from build123d import *

# Parameters (mm, degrees)
SKETCH1_R           = 1.5875
SKETCH1_R_2         = 1.905
SKETCH1_R_3         = 13.5001
BOSS_EXTRUDE1_DEPTH = 6.35


with BuildPart() as part:
    # Sketch1 → Boss-Extrude1 (new body)
    with BuildSketch(Plane.XY):
        with BuildLine():
            ThreePointArc((17.78, 25.4), (18.678025612, 25.028025612), (19.05, 24.13))
            Line((19.05, 24.13), (19.05, 0))
            ThreePointArc((19.05, 0), (13.470384182, -13.470384182), (0, -19.05))
            Line((0, -19.05), (-26.67, -19.05))
            ThreePointArc((-26.67, -19.05), (-67.081152545, -2.311152545), (-83.82, 38.1))
            ThreePointArc((-83.82, 38.1), (-81.588153673, 43.488153673), (-76.2, 45.72))
            Line((-76.2, 45.72), (-50.8, 45.72))
            ThreePointArc((-50.8, 45.72), (-47.214117647, 44.823529412), (-44.471972318, 42.345051903))
            ThreePointArc((-44.471972318, 42.345051903), (-30.704117647, 29.901029412), (-12.7, 25.4))
            Line((-12.7, 25.4), (17.78, 25.4))
        make_face()
        with Locations((-7.750175, 13.423696868)):
            Circle(SKETCH1_R, mode=Mode.SUBTRACT)
        with Locations((-13.423696868, 7.750175)):
            Circle(SKETCH1_R, mode=Mode.SUBTRACT)
        with Locations((-15.50035, 0)):
            Circle(SKETCH1_R, mode=Mode.SUBTRACT)
        with Locations((-13.423696868, -7.750175)):
            Circle(SKETCH1_R, mode=Mode.SUBTRACT)
        with Locations((-7.750175, -13.423696868)):
            Circle(SKETCH1_R, mode=Mode.SUBTRACT)
        with Locations((0, -15.50035)):
            Circle(SKETCH1_R, mode=Mode.SUBTRACT)
        with Locations((7.750175, -13.423696868)):
            Circle(SKETCH1_R, mode=Mode.SUBTRACT)
        with Locations((13.423696868, -7.750175)):
            Circle(SKETCH1_R, mode=Mode.SUBTRACT)
        with Locations((15.50035, 0)):
            Circle(SKETCH1_R, mode=Mode.SUBTRACT)
        with Locations((13.423696868, 7.750175)):
            Circle(SKETCH1_R, mode=Mode.SUBTRACT)
        with Locations((7.750175, 13.423696868)):
            Circle(SKETCH1_R, mode=Mode.SUBTRACT)
        with Locations((0, 15.50035)):
            Circle(SKETCH1_R, mode=Mode.SUBTRACT)
        with Locations((-50.8, 38.1)):
            Circle(SKETCH1_R_2, mode=Mode.SUBTRACT)
        with Locations((-76.2, 38.1)):
            Circle(SKETCH1_R_2, mode=Mode.SUBTRACT)
        Circle(SKETCH1_R_3, mode=Mode.SUBTRACT)
    extrude(amount=BOSS_EXTRUDE1_DEPTH)


solid = part.part
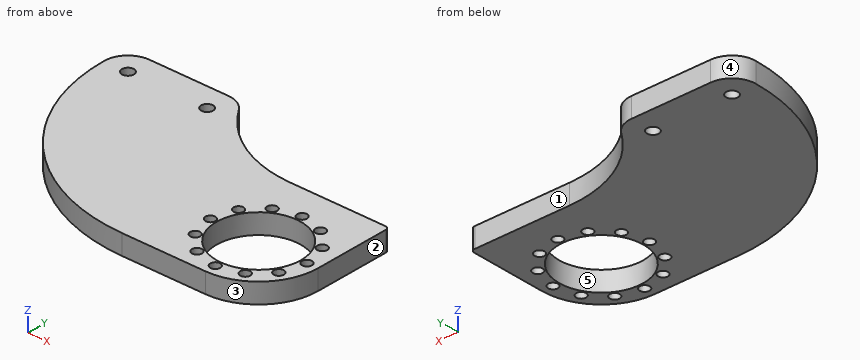
Model file for the job. Use its own axes, mm. Face numbers are marked on the shaded views. A direction names the side the tool comes from. Coordinates: 2 decimals unless noted, no trailing zeros. Write each loop counter-clockwise with the first axis right and the second up, starting at its lowest first coordinate (ties: lowest second). Pieces come first, ordered by that corner, then holes. Notation, with made-up numbers: (48.25, -33.5) -> (83.25, -33.5) arc R19 ccw to (83.25, -28.5) -> close; hole circle Ø5 at (-2, 2.25). An arc over 180 degrees is marked (long way). One line per item, written item: value. Start each with the question number.
1) Pull direction X, two halves, no side cores. Call the marked faces 3, 4 and 5: +X half, -X half, draft (parallel to the pull), parting line (faces both ways), or undercut.
2) Probe probe 1 along Y at (x, z) = (-7, 5.5); probe 2 along Y at (x, z) = (-1, 3.75); probe 3 along X at (y, z) = (38, 5). List the from-to ranges inside material, lowest first.
3) Slice it at C-C on y = 19.5. Write the cut outline in (x, z).
4) Slice it at B-B on z = 2.5. Count the separate pieces of the cut face and the enclosed holes in it, then the cut area to 3 significant figures.
5) Which spindle directions (+Z, -Z, +X, -X, +Y, -Y) get a long thin tool onto all of the face, cutting with end or side? Do the marked faces 1 and 2. Say none if no direction does.
6) Flat gauge pins, fed straight in: pin 1 Ø2 at (y, z) = (-7, 3.5) entering from -X; pin 2 Ø24.5 at (x, y) = (0, 0) entering from -Z; pin 3 Ø3 at (x, z) = (5, 3) entering from +Y. Where does each tip first touch, or does it go through?
7) Slice it at A-A on x = 5. Write the cut outline in (y, z).
8) Slice it at D-D on x = -61. Write the cut outline in (y, z).
Answers follow:
1. face 3: +X half
1. face 4: -X half
1. face 5: undercut
2. probe 1: -19.05 to -14.82, -12.02 to -11.54, 11.54 to 12.02, 14.82 to 25.4
2. probe 2: -19.05 to -16.73, -14.27 to -13.46, 13.46 to 14.27, 16.73 to 25.4
2. probe 3: -83.82 to -78.1, -74.3 to -52.7, -48.9 to -41.08
3. outline: (-80.71, 0) -> (19.05, 0) -> (19.05, 6.35) -> (-80.71, 6.35) -> close
4. separate pieces: 1
4. enclosed holes: 15
4. area: 4,040 mm2
5. face 1: +Z, -Z, +X, +Y
5. face 2: +Z, -Z, +X, +Y, -Y
6. pin 1: x = -63.02
6. pin 2: through
6. pin 3: y = 25.4
7. outline: (-18.38, 0) -> (-12.54, 0) -> (-12.54, 6.35) -> (-18.38, 6.35) -> close; (12.54, 0) -> (25.4, 0) -> (25.4, 6.35) -> (12.54, 6.35) -> close
8. outline: (-7.59, 0) -> (45.72, 0) -> (45.72, 6.35) -> (-7.59, 6.35) -> close
